The listing builds one solid part. Answer for the finished solid, in the listing's coordinates (mm). A direction names the side the tool comes from. Give positions to 0.01 mm unless a question says otherwise; leave off trailing zeros. Order: outer loops, then holes, each group sorted by start corner. A loop starts at its lowest first (then second) coordinate and runs counter-clockwise, first axis right, second up.
```python
from build123d import *
from build123d.topology import SkipClean

# Parameters (mm, degrees)
SCHIZZO1_R                   = 29.1
SCHIZZO1_R_2                 = 26.1
ESTRUSIONE_ESTRUSIONE1_DEPTH = 20
SCHIZZO2_W                   = 5
SCHIZZO2_H                   = 17.200297627
ESTRUSIONE_ESTRUSIONE2_DEPTH = 20
SCHIZZO3_W                   = 30
SCHIZZO3_H                   = 16.910350343
TAGLIO_ESTRUSIONE1_DEPTH     = 51.426282829
TAGLIO_ESTRUSIONE3_DEPTH     = 51.426282829
SCHIZZO5_R                   = 1.75
TAGLIO_ESTRUSIONE4_DEPTH     = 65.084397477
SCHIZZO6_R                   = 3.25
TAGLIO_ESTRUSIONE5_DEPTH     = 2
TAGLIO_ESTRUSIONE6_DEPTH     = 2
ESTRUSIONE_ESTRUSIONE3_START = -5
ESTRUSIONE_ESTRUSIONE3_DEPTH = 10
ESTRUSIONE_ESTRUSIONE4_START = 5
SCHIZZO10_W                  = 81.6
SCHIZZO10_H                  = 5
ESTRUSIONE_ESTRUSIONE4_DEPTH = 20
SCHIZZO9_R                   = 2
TAGLIO_ESTRUSIONE7_DEPTH     = 103.305913808


with BuildPart() as part:
    # Schizzo1 → Estrusione-Estrusione1 (new body)
    with BuildSketch(Plane.XY):
        Circle(SCHIZZO1_R)
        Circle(SCHIZZO1_R_2, mode=Mode.SUBTRACT)
    extrude(amount=ESTRUSIONE_ESTRUSIONE1_DEPTH)

    # Schizzo2 → Estrusione-Estrusione2 (add)
    with BuildSketch(Plane.XY.offset(20)):
        with Locations((-17.5, 27.399851187)):
            Rectangle(SCHIZZO2_W, SCHIZZO2_H)
        with Locations((17.5, 27.399851187)):
            Rectangle(SCHIZZO2_W, SCHIZZO2_H)
    extrude(amount=-ESTRUSIONE_ESTRUSIONE2_DEPTH)

    # Schizzo3 → Taglio-Estrusione1 (cut, through all)
    with BuildSketch(Plane.XY.offset(20)):
        with Locations((0, 27.544824829)):
            Rectangle(SCHIZZO3_W, SCHIZZO3_H)
    extrude(amount=-TAGLIO_ESTRUSIONE1_DEPTH, mode=Mode.SUBTRACT)

    # Schizzo4 → Taglio-Estrusione3 (cut, through all)
    with SkipClean():  # the faces are left unmerged after this step: merging them gives an invalid solid
        with BuildSketch(Plane.XY.offset(20)):
            with BuildLine():
                Line((-15, 18.799702373), (-18.104728407, 18.799702373))
                ThreePointArc((-18.104728407, 18.799702373), (-10.214611803, -24.01815367), (26.1, 0))
                ThreePointArc((26.1, 0), (24.01815367, 10.214611803), (18.104728407, 18.799702373))
                Line((18.104728407, 18.799702373), (15, 18.799702373))
                Line((15, 18.799702373), (15, 21.359073014))
                ThreePointArc((15, 21.359073014), (0, 26.1), (-15, 21.359073014))
                Line((-15, 21.359073014), (-15, 18.799702373))
            make_face()
            with BuildLine():
                ThreePointArc((-15, 21.359073014), (-16.601757595, 20.139305965), (-18.104728407, 18.799702373))
                Line((-18.104728407, 18.799702373), (-15, 18.799702373))
                Line((-15, 18.799702373), (-15, 21.359073014))
            make_face()
            with BuildLine():
                Line((15, 18.799702373), (18.104728407, 18.799702373))
                ThreePointArc((18.104728407, 18.799702373), (16.601757595, 20.139305965), (15, 21.359073014))
                Line((15, 21.359073014), (15, 18.799702373))
            make_face()
        extrude(amount=-TAGLIO_ESTRUSIONE3_DEPTH, mode=Mode.SUBTRACT)

    # Schizzo5 → Taglio-Estrusione4 (cut, through all)
    with SkipClean():  # the faces are left unmerged after this step: merging them gives an invalid solid
        with BuildSketch(Plane.ZY.offset(20)):
            with Locations((10, 31)):
                Circle(SCHIZZO5_R)
        extrude(amount=-TAGLIO_ESTRUSIONE4_DEPTH, mode=Mode.SUBTRACT)

    # Schizzo6 → Taglio-Estrusione5 (cut)
    with SkipClean():  # the faces are left unmerged after this step: merging them gives an invalid solid
        with BuildSketch(Plane.ZY.offset(20)):
            with Locations((10, 31)):
                Circle(SCHIZZO6_R)
        extrude(amount=-TAGLIO_ESTRUSIONE5_DEPTH, mode=Mode.SUBTRACT)

    # Schizzo7 → Taglio-Estrusione6 (cut)
    with SkipClean():  # the faces are left unmerged after this step: merging them gives an invalid solid
        with BuildSketch(Plane(origin=(20, 0, 0), x_dir=(0, 0, -1), z_dir=(1, 0, 0))):
            Polygon((-8.41228676, 28.25), (-6.824573519, 31), (-8.41228676, 33.75), (-11.58771324, 33.75), (-13.175426481, 31), (-11.58771324, 28.25), align=None)
        extrude(amount=-TAGLIO_ESTRUSIONE6_DEPTH, mode=Mode.SUBTRACT)

    # Schizzo8 → Estrusione-Estrusione3 (add)
    with SkipClean():  # the faces are left unmerged after this step: merging them gives an invalid solid
        with BuildSketch(Plane(origin=(0, 0, 0), x_dir=(-1, 0, 0), z_dir=(0, 0, -1)).offset(ESTRUSIONE_ESTRUSIONE3_START)):
            with BuildLine():
                Line((-52.5, -49.5), (-52.5, -54.5))
                Line((-52.5, -54.5), (29.1, -54.5))
                Line((29.1, -54.5), (29.1, 0))
                ThreePointArc((29.1, 0), (-1.93856651, -29.035357065), (-28.841715456, 3.868520332))
                Line((-28.841715456, 3.868520332), (-36, -49.5))
                Line((-36, -49.5), (-52.5, -49.5))
            make_face()
            with BuildLine():
                ThreePointArc((-28.841715456, 3.868520332), (-1.93856651, -29.035357065), (29.1, 0))
                Line((29.1, 0), (26.099231032, 0.2003485))
                ThreePointArc((26.099231032, 0.2003485), (-1.738714293, -26.042021285), (-25.840946488, 3.668171832))
                Line((-25.840946488, 3.668171832), (-28.841715456, 3.868520332))
            make_face()
        extrude(amount=-ESTRUSIONE_ESTRUSIONE3_DEPTH)

    # Schizzo10 → Estrusione-Estrusione4 (add)
    with SkipClean():  # the faces are left unmerged after this step: merging them gives an invalid solid
        with BuildSketch(Plane(origin=(0, 0, 5), x_dir=(-1, 0, 0), z_dir=(0, 0, -1)).offset(ESTRUSIONE_ESTRUSIONE4_START)):
            with Locations((-11.7, -52)):
                Rectangle(SCHIZZO10_W, SCHIZZO10_H)
        extrude(amount=-ESTRUSIONE_ESTRUSIONE4_DEPTH)

    # Schizzo9 → Taglio-Estrusione7 (cut, through all)
    with SkipClean():  # the faces are left unmerged after this step: merging them gives an invalid solid
        with BuildSketch(Plane(origin=(0, -49.5, 0), x_dir=(1, 0, 0), z_dir=(0, 1, 0))):
            with Locations(Location((47.5, -10, 0), (0, 0, 270))):
                Circle(SCHIZZO9_R)
        extrude(amount=-TAGLIO_ESTRUSIONE7_DEPTH, mode=Mode.SUBTRACT)


solid = part.part
```
1) Find section D-D (x = 0). Write down the section's boundary in (y, z), then the cut area to 3 significant figures.
Geometry says:
outline: (-54.5, 0) - (-49.5, 0) - (-49.5, 5) - (-29.1, 5) - (-29.1, 0) - (-26.1, 0) - (-26.1, 20) - (-29.1, 20) - (-29.1, 15) - (-49.5, 15) - (-49.5, 20) - (-54.5, 20) - close
area: 364 mm2
2) For a pull along Y with two mould halves and no side action, classify faces 1 (the flat face through (19, 33.75, 10)), 2 (the flat face through (-24, 11, 20)) as +Y half, -Y half, draft (parallel to the pull), parting line (faces both ways), or undercut.
Geometry says:
face 1: undercut
face 2: draft
3) Straight lines are drawn through the part: probe 1 along X at (y, z) = (26.5, 16.5); probe 2 along Y at (x, z) = (18, 15.5); probe 3 along X at (y, z) = (-53.15, 10). For each, find the intervals that lie inside material, in ascending order.
Geometry says:
probe 1: x = -20 to -15, 15 to 20
probe 2: y = -54.5 to -49.5, -22.87 to -18.9, 18.9 to 36
probe 3: x = -29.1 to 45.5, 49.5 to 52.5
4) Find section C-C (z = 10). Count the separate pieces of the cut face and the enclosed holes in it, then the cut area to 3 significant figures.
Geometry says:
separate pieces: 4
enclosed holes: 0
area: 2,620 mm2
5) Find section B-B (y = -14). Write down the section's boundary in (x, z), then the cut area to 3 significant figures.
Geometry says:
outline: (-29.1, 5) - (-25.51, 5) - (-25.51, 0) - (-22.03, 0) - (-22.03, 20) - (-25.51, 20) - (-25.51, 15) - (-29.1, 15) - close; (22.03, 0) - (25.51, 0) - (25.51, 5) - (31.24, 5) - (31.24, 15) - (25.51, 15) - (25.51, 20) - (22.03, 20) - close
area: 233 mm2
6) A tool of negligible diameter and unlimited length cuts with its end or side. For faces 3 (the flat face through (4, -34, 15)), 4 (the flat face through (19.014, 32.394, 12.37)), 5 (the flat face through (20, 27, 10)), from which of +Z, -Z, +X, -X, +Y, -Y can it reach the whole face along a straight path? Write none if from no direction.
Geometry says:
face 3: +Z
face 4: +X
face 5: +Z, -Z, +X, +Y
7) Given P1, Ø8.5, axis at y = 31, z = 10, coming from the -X side; P2, Ø4.5, axis at y = 28.5, z = 8, coming from the +X side; P3, Ø4.5, axis at y = 31, z = 10, coming from the +X side; P4, Ø2.5, axis at x = 47.5, z = 10, coming from the +Y side, each flat-ended and moving along its own axis, determine where each tip first touches the part or whether it passes through.
Geometry says:
P1: stops at x = -20
P2: stops at x = 20
P3: stops at x = 18
P4: passes through
8) Find section A-A (x = 16). Write down the section's boundary in (y, z), then the cut area to 3 significant figures.
Geometry says:
outline: (-54.5, 0) - (-49.5, 0) - (-49.5, 5) - (-24.31, 5) - (-24.31, 0) - (-20.62, 0) - (-20.62, 20) - (-24.31, 20) - (-24.31, 15) - (-49.5, 15) - (-49.5, 20) - (-54.5, 20) - close; (20.62, 0) - (36, 0) - (36, 20) - (20.62, 20) - close; hole circle Ø3.5 at (31, 10)
area: 724 mm2
